Part print with two shaded views. Sizes in mm from the minimum x, y, z corner. A direction names the side the tool comes from. Give positions to 0.01 mm unless a question says otherwise; leave off trailing zeros. Order: outer loops, then holes, each group sorted by start corner. A loop starts at its lowest first (then second) coordinate and runs counter-clockwise, first axis right, second up. Notation, with made-up numbers: M -5.5,20 L 8.5,20 A10 ccw 8.5,38 Z; hole C 50,87 d2. An arc over 180 degrees is marked long. Answer as CSV lines item,"result".
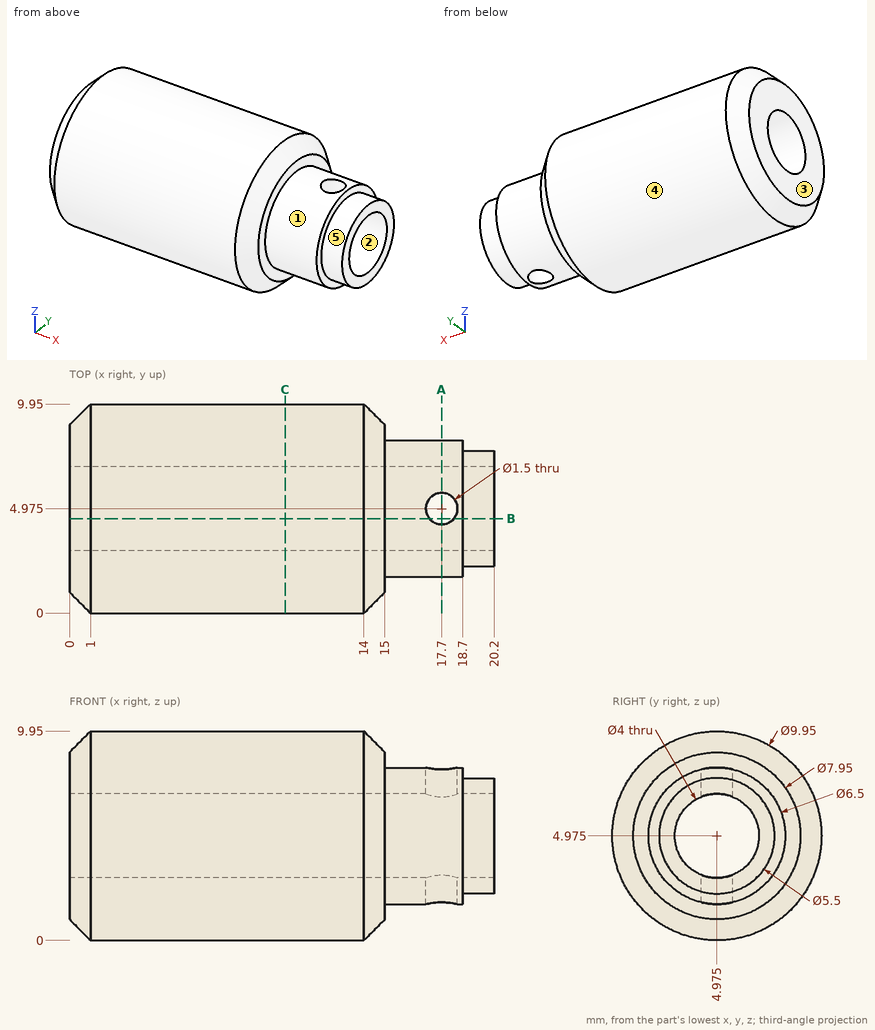
Item 1: Pull direction Y, two halves, no side cores. Call the marked faces 1, 2 and 3: released by +Y, released by -Y, zero draft, split by the parting line, or undercut.
Geometry says:
face 1,"split by the parting line"
face 2,"undercut"
face 3,"zero draft"
Item 2: Band-saw the part on A-A (x = 17.7). Give the cut face in (y, z) (3 decimals).
Geometry says:
outline,"M 4.225,1.813 L 4.225,3.121 A2 cw 4.225,6.829 L 4.225,8.137 A3.25 ccw Z; M 5.725,1.813 A3.25 ccw 5.725,8.137 L 5.725,6.829 A2 cw 5.725,3.121 Z"
Item 3: Probe line 1 along Z through (x, y) = (10.25, 5); line 2 along Z through (x, y) = (19.25, 3.75); line 3 along Y through (x, z) = (18, 6). List the from-to ranges inside material, lowest first. Write a range as from..to.
Geometry says:
line 1,"z = 0..2.98, 6.97..9.95"
line 2,"z = 2.51..3.39, 6.56..7.44"
line 3,"y = 1.89..3.26, 6.69..8.06"
Item 4: Drop flat-ended pins along their axis: pin 1 (1.7 mm diameter, centred on x = 17.7, y = 4.975, fed in from -Z) (3 decimals); pin 2 (1 mm diameter, centred on x = 13.5, z = 8, fed in from +Y); pin 3 (1.4 mm diameter, centred on x = 17.7, y = 4.975, fed in from +Z). Give the stop position or say it passes through.
Geometry says:
pin 1,"stops at z = 1.725"
pin 2,"stops at y = 9.26"
pin 3,"passes through"
Item 5: Band-saw the part on B-B (y = 4.5). State how many separate pieces and enclosed holes the cut face has, and give its area (3 significant figures).
Geometry says:
separate pieces,"4"
enclosed holes,"0"
area,"97.0 mm2"
Item 6: Band-saw the part on C-C (x = 10.25). Give the cut face in (y, z) (3 decimals), and give its area (3 significant figures).
Geometry says:
outline,"C 4.975,4.975 d9.95; hole C 4.975,4.975 d4"
area,"65.2 mm2"
Item 7: 3-axis set-ups, long thin cutter, end or side, ignore diameter. For the marked faces 4 and 5: which of +Z, -Z, +X, -X, +Y, -Y reach the whole face in a straight line?
Geometry says:
face 4,"+X, -X"
face 5,"+X"
